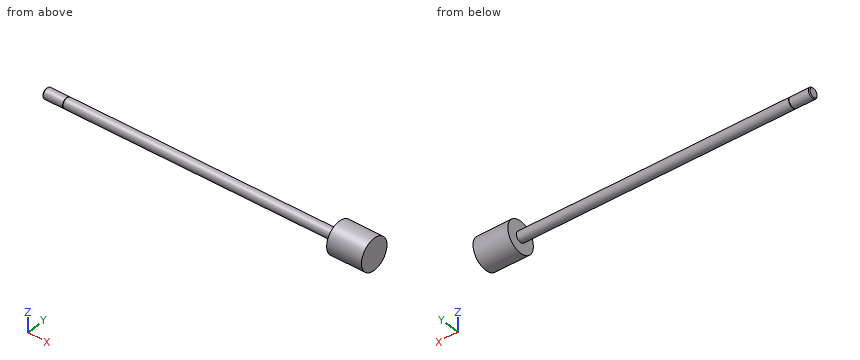
Autodesk Inventor part; units mm, degrees
ref_plane "dia1_XY" through (0, 3.175, 0) normal (1, 0, 0) x (0, 0, -1)
ref_plane "dia1_YZ" through (0, 3.175, 0) normal (0, 0, -1) x (0, 1, 0)
ref_plane "dia1_ZX" through (0, 3.175, 0) normal (0, 1, 0) x (1, 0, 0)
sketch "Sketch_1" plane through (0, 0, 0) normal (0, 0, 1) x (1, 0, 0)
  line L0 (188.9252, 0) -> (0, 0)
  line L1 (0, 0) -> (0, 3.175)
  line L2 (0, 3.175) -> (167.4876, 3.175)
  line L3 (167.4876, 3.175) -> (167.4876, 9.6203)
  line L4 (167.4876, 9.6203) -> (188.9252, 9.6203)
  line L5 (188.9252, 9.6203) -> (188.9252, 0)
  line L6 (188.9252, 0) -> (0, 0)
revolve "Revolution1" add sketch "Sketch_1" angle 360 about axis through (188.9252, 0, 0) along (1, 0, 0)
sketch "Sketch_3" plane through (0, 0, 0) normal (0, 0, 1) x (1, 0, 0)
  line L0 (0, 0) -> (-12.7, 0)
  line L1 (-12.7, 0) -> (-12.7, 2.634)
  line L2 (-12.7, 2.634) -> (-12.159, 3.175)
  line L3 (-12.159, 3.175) -> (0, 3.175)
  line L4 (0, 3.175) -> (0, 0)
  line L5 (0, 0) -> (-12.7, 0)
revolve "Revolution2" add sketch "Sketch_3" angle 360 about axis through (0, 0, 0) along (1, 0, 0)
thread "Thread1"
sketch "Sketch_30" plane through (0, 0, 0) normal (0, 0, 1) x (1, 0, 0)
  line L0 (0, 0) -> (-0.254, 0)
  line L1 (-0.254, 2.921) -> (0, 2.921)
  line L2 (0, 2.921) -> (0, 3.429)
  line L3 (0, 3.429) -> (-0.254, 3.429)
  line L4 (-0.254, 3.429) -> (-0.254, 2.921)
revolve "Revolution3" cut sketch "Sketch_30" angle 360 about axis through (0, 0, 0) along (1, 0, 0)
ref_plane "dia1_XY" through (0, 3.175, 0) normal (1, 0, 0) x (0, 0, -1)
ref_plane "dia1_YZ" through (0, 3.175, 0) normal (0, 0, -1) x (0, 1, 0)
ref_plane "dia1_ZX" through (0, 3.175, 0) normal (0, 1, 0) x (1, 0, 0)
ref_plane "dia12_XY" through (0, 0, 10.9537) normal (1, 0, 0) x (0, 0, -1)
ref_plane "dia12_YZ" through (0, 0, 10.9537) normal (0, 0, -1) x (0, 1, 0)
ref_plane "dia12_ZX" through (0, 0, 10.9537) normal (0, 1, 0) x (1, 0, 0)
ref_plane "dia2_XY" through (0, -3.175, 0) normal (1, 0, 0) x (0, 0, -1)
ref_plane "dia2_YZ" through (0, -3.175, 0) normal (0, 0, -1) x (0, 1, 0)
ref_plane "dia2_ZX" through (0, -3.175, 0) normal (0, 1, 0) x (1, 0, 0)
ref_plane "dia22_XY" through (0, 0, -10.9537) normal (1, 0, 0) x (0, 0, -1)
ref_plane "dia22_YZ" through (0, 0, -10.9537) normal (0, 0, -1) x (0, 1, 0)
ref_plane "dia22_ZX" through (0, 0, -10.9537) normal (0, 1, 0) x (1, 0, 0)
ref_plane "rl1_XY" through (-12.7, 0, 0) normal (1, 0, 0) x (0, 0, -1)
ref_plane "rl1_YZ" through (-12.7, 0, 0) normal (0, 0, -1) x (0, 1, 0)
ref_plane "rl1_ZX" through (-12.7, 0, 0) normal (0, 1, 0) x (1, 0, 0)
ref_plane "rl2_XY" through (0, 0, 0) normal (1, 0, 0) x (0, 0, -1)
ref_plane "rl2_YZ" through (0, 0, 0) normal (0, 0, -1) x (0, 1, 0)
ref_plane "rl2_ZX" through (0, 0, 0) normal (0, 1, 0) x (1, 0, 0)
ref_plane "rod_cp_XY" through (0, 0, 0) normal (1, 0, 0) x (0, 0, -1)
ref_plane "rod_cp_YZ" through (0, 0, 0) normal (0, 0, -1) x (0, 1, 0)
ref_plane "rod_cp_ZX" through (0, 0, 0) normal (0, 1, 0) x (1, 0, 0)
ref_plane "thd1_XY" through (-12.7, 3.175, 0) normal (1, 0, 0) x (0, 0, -1)
ref_plane "thd1_YZ" through (-12.7, 3.175, 0) normal (0, 0, -1) x (0, 1, 0)
ref_plane "thd1_ZX" through (-12.7, 3.175, 0) normal (0, 1, 0) x (1, 0, 0)
ref_plane "thd2_XY" through (-12.7, -3.175, 0) normal (1, 0, 0) x (0, 0, -1)
ref_plane "thd2_YZ" through (-12.7, -3.175, 0) normal (0, 0, -1) x (0, 1, 0)
ref_plane "thd2_ZX" through (-12.7, -3.175, 0) normal (0, 1, 0) x (1, 0, 0)
ref_plane "to_rod_clevis_XY" through (-16.764, 0, 0) normal (1, 0, 0) x (0, 0, -1)
ref_plane "to_rod_clevis_YZ" through (-16.764, 0, 0) normal (0, 0, -1) x (0, 1, 0)
ref_plane "to_rod_clevis_ZX" through (-16.764, 0, 0) normal (0, 1, 0) x (1, 0, 0)
properties part number "C-045-DP0_rod" material "Steel, Galvanized"
Read the model definition and answer for the solid it produces. Units are mm, in the model's axes. Coordinates: 2 decimals unless noted, no trailing zeros. Order: outer loops, then holes, each group sorted by start corner. A loop starts at its lowest first (then second) coordinate and runs counter-clockwise, first axis right, second up. Notation, with made-up numbers: M -11,28 L 43,28 A19 ccw 43,35 Z; hole C 0.5,-28 d10. An arc over 180 degrees is marked long. Put each result on its own line as item: value. Start each with the question number.
Item 1: Section A-A, the plane z = 0 is taken. Determine the outline of the cut face in (x, y) (3 decimals).
Item 2: Consider probe 1 along X at (y, z) = (3.5, -1); probe 2 along Z at (x, y) = (65, -0.5); probe 3 along Y at (x, z) = (5.5, -1.25). Determine where each line is inside the solid, lowest interval first. Write a range as [from, to].
Item 3: Section C-C, the plane x = 122 is taken. Determine the outline of the cut face in (y, z) (3 decimals), plus the area to 3 significant figures.
Item 4: Section D-D, the plane y = 7.5 is taken. Determine the outline of the cut face in (x, z), plus the area to 3 significant figures.
Item 5: Given pin 1 Ø6 at (x, z) = (87.5, -1.5) entering from -Y (3 decimals); pin 2 Ø4 at (y, z) = (-3.5, 5) entering from -X; pin 3 Ø1 at (x, z) = (26.5, -1) entering from +Y, each flat-ended and moving along its own axis, determine where each tip first touches the part or whether it passes through.
Computed:
1. outline: M -12.7,-2.634 L -12.159,-3.175 L -0.254,-3.175 L -0.254,-2.921 L 0,-2.921 L 0,-3.175 L 167.488,-3.175 L 167.488,-9.62 L 188.925,-9.62 L 188.925,9.62 L 167.488,9.62 L 167.488,3.175 L 0,3.175 L 0,2.921 L -0.254,2.921 L -0.254,3.175 L -12.159,3.175 L -12.7,2.634 Z
2. probe 1: x = [167.49, 188.93]
2. probe 2: z = [-3.14, 3.14]
2. probe 3: y = [-2.92, 2.92]
3. outline: C 0,0 d6.35
3. area: 31.7 mm2
4. outline: M 167.49,-6.02 L 188.93,-6.02 L 188.93,6.02 L 167.49,6.02 Z
4. area: 258 mm2
5. pin 1: stops at y = -3.175
5. pin 2: stops at x = 167.49
5. pin 3: stops at y = 3.14
